Check sheet for the drawn part. Datum: minimum x, y, z corner. Units: mm. Round coordinates to 2 decimals unless told otherwise and drop trailing zeros. Write each loop counter-clockwise with the first axis right and the second up, starting at its lowest first coordinate (ties: lowest second). Pieces come first, ordered by that corner, then holes. Notation, with made-up numbers: M 19.25,80 L 71.25,80 A29 cw 71.25,110 Z; hole C -11.75,0.5 d3. An arc over 180 degrees is marked long. Put each result on its own line as item: value.
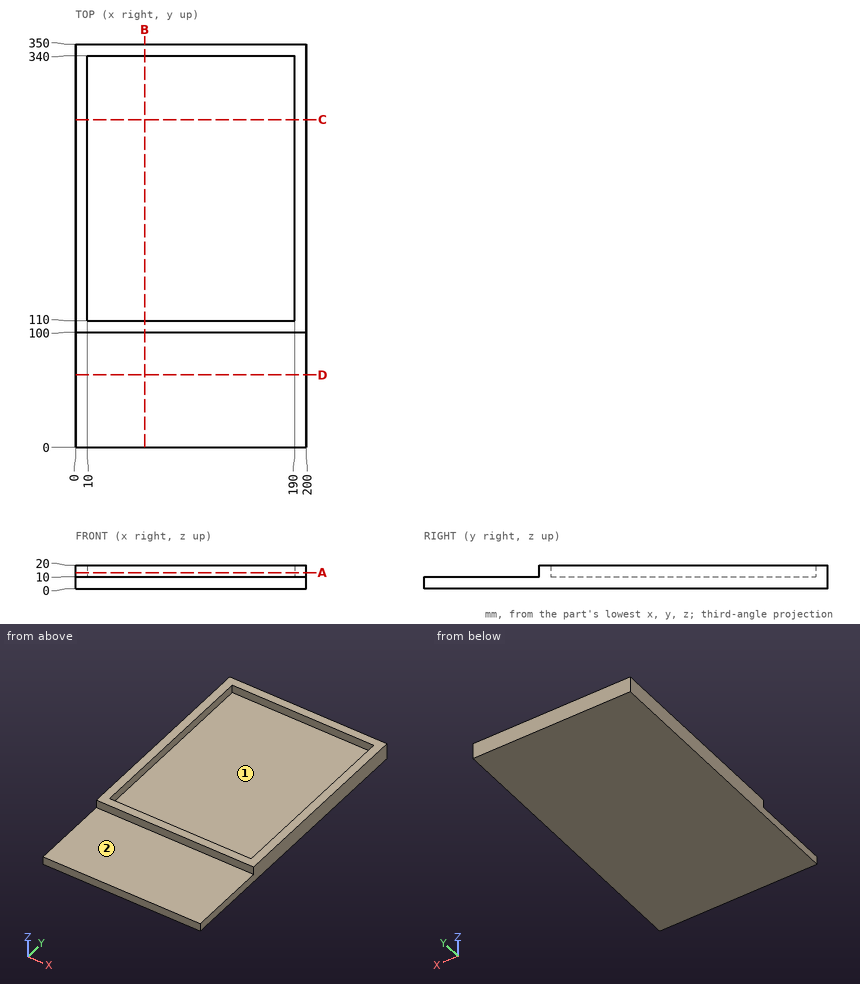
1. Cross-section at B-B (x = 60). Enter the section's corners in (y, z).
Computed values:
outline: M 0,0 L 350,0 L 350,20 L 340,20 L 340,10 L 110,10 L 110,20 L 100,20 L 100,10 L 0,10 Z
2. Scan lines: probe 1 along Y at (x, z) = (30.5, 12); probe 2 along Z at (x, y) = (129.5, 64); probe 3 along X at (y, z) = (267, 17.75). Record each from-to range of solid material in increasing order.
Computed values:
probe 1: y = 100 to 110, 340 to 350
probe 2: z = 0 to 10
probe 3: x = 0 to 10, 190 to 200
3. Cross-section at C-C (y = 284.5). Enter the section's corners in (x, z).
Computed values:
outline: M 0,0 L 200,0 L 200,20 L 190,20 L 190,10 L 10,10 L 10,20 L 0,20 Z
4. Cross-section at D-D (y = 63). Enter the section's corners in (x, z), then the cut area to 3 significant figures.
Computed values:
outline: M 0,0 L 200,0 L 200,10 L 0,10 Z
area: 2,000 mm2
5. Release check for a two-part mould opening along Y. For the marked faces 1 and 2 record: +Y half, -Y half, draft (parallel to the pull), parting line (faces both ways), or undercut.
Computed values:
face 1: undercut
face 2: draft
6. Depth check by flat-ended pin: pin 1 Ø5 at (x, z) = (117, 16) entering from -Y; pin 2 Ø5 at (x, y) = (144, 201.5) entering from +Z. Enter the tip coordinate at first touch or a pass-through.
Computed values:
pin 1: stops at y = 100
pin 2: stops at z = 10
7. Cross-section at A-A (z = 13.75). Enter the section's corners in (x, y).
Computed values:
outline: M 0,100 L 200,100 L 200,350 L 0,350 Z; hole M 10,110 L 190,110 L 190,340 L 10,340 Z
